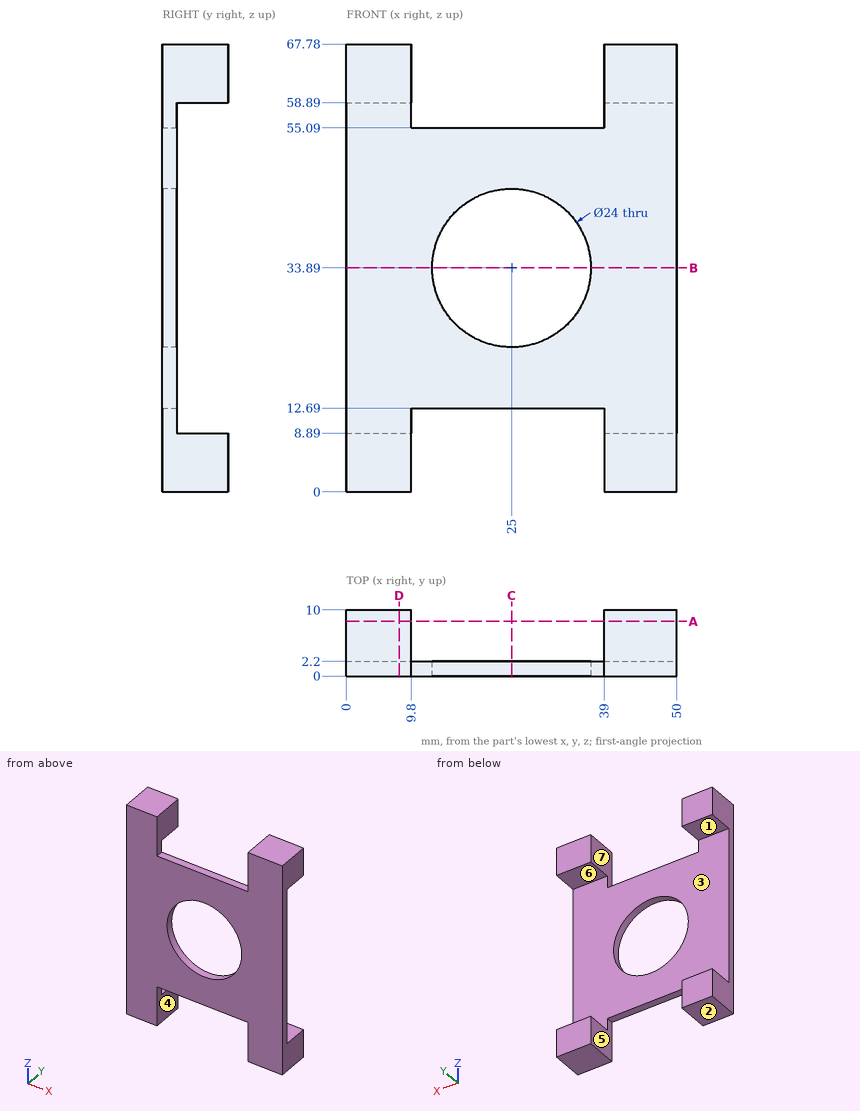
Answer from the drawing. Dimensions are ordinates in mm from the lowest x, y and z of the part. A direction names the side the tool comes from. Give positions to 0.01 mm unless a question says otherwise; leave off trailing zeros. Write each loop counter-clockwise with the first axis right and the second up, starting at its lowest first coordinate (ties: lowest second). Pieces come first, ordered by that corner, then holes. Notation, with made-up numbers: (13, 36.5) - (68, 36.5) arc R12 ccw to (68, 47.5) - close; hole circle Ø11 at (27.5, 51). An arc over 180 degrees is marked (long way). Answer in a Markdown table with one row per item. Add a question column.
Item 1: Section B-B, the plane z = 33.89 is taken. Write down the section's boundary in (x, y), and give its area (3 significant figures).
Item 2: Determine the mould class of the marked faces 1, 2, 3 and 4 for opening direction Z: pulls with the +Z half, pulls with the -Z half, needs draft (parallel to the pull), parting line crosses it, or undercut.
Item 3: Section C-C, the plane x = 25 is taken. Write down the section's boundary in (y, z), and give its area (3 significant figures).
Item 4: Section D-D, the plane x = 8 is taken. Write down the section's boundary in (y, z).
Item 5: Find the intervals of material crossed by L1, parallel to Z at x = 25, y = 0.75; L2, parallel to Z at x = 7.5, y = 9.5; L3, parallel to X at y = 8.75, z = 62, in increasing order.
Item 6: Flat-ended cylindrical pins translate along their axes: P1, Ø1.8, axis at x = 27, y = 0.5, coming from the -Z side; P2, Ø2, axis at x = 23.5, z = 44, coming from the -Y side; P3, Ø1.1, axis at x = 28, y = 1, coming from the +Z side. Find the tip coordinate at first contact, or state that the pin passes through.
Item 7: A tool of negligible diameter and unlimited length cuts with its end or side. For the marked faces 5, 6 and 7, from which of +Z, -Z, +X, -X, +Y, -Y can it reach the whole face along a straight path? Write none if from no direction.
Item 8: Section A-A, the plane y = 8.25 is taken. Write down the section's boundary in (x, z).
Recorded:
| question | item | result |
|---|---|---|
| 1 | outline | (0, 0) - (13, 0) - (13, 2.2) - (0, 2.2) - close; (37, 0) - (50, 0) - (50, 2.2) - (37, 2.2) - close |
| 1 | area | 57.2 mm2 |
| 2 | face 1 | undercut |
| 2 | face 2 | pulls with the -Z half |
| 2 | face 3 | undercut |
| 2 | face 4 | needs draft |
| 3 | outline | (0, 12.69) - (2.2, 12.69) - (2.2, 21.89) - (0, 21.89) - close; (0, 45.89) - (2.2, 45.89) - (2.2, 55.09) - (0, 55.09) - close |
| 3 | area | 40.5 mm2 |
| 4 | outline | (0, 0) - (10, 0) - (10, 8.89) - (2.2, 8.89) - (2.2, 58.89) - (10, 58.89) - (10, 67.78) - (0, 67.78) - close |
| 5 | L1 | z = 12.69 to 21.89, 45.89 to 55.09 |
| 5 | L2 | z = 0 to 8.89, 58.89 to 67.78 |
| 5 | L3 | x = 0 to 9.8, 39 to 50 |
| 6 | P1 | stops at z = 12.69 |
| 6 | P2 | passes through |
| 6 | P3 | stops at z = 55.09 |
| 7 | face 5 | -Z, +Y, -Y |
| 7 | face 6 | +X, -X, +Y |
| 7 | face 7 | +Z, +Y, -Y |
| 8 | outline | (0, 0) - (9.8, 0) - (9.8, 8.89) - (0, 8.89) - close; (0, 58.89) - (9.8, 58.89) - (9.8, 67.78) - (0, 67.78) - close; (39, 0) - (50, 0) - (50, 8.89) - (39, 8.89) - close; (39, 58.89) - (50, 58.89) - (50, 67.78) - (39, 67.78) - close |
